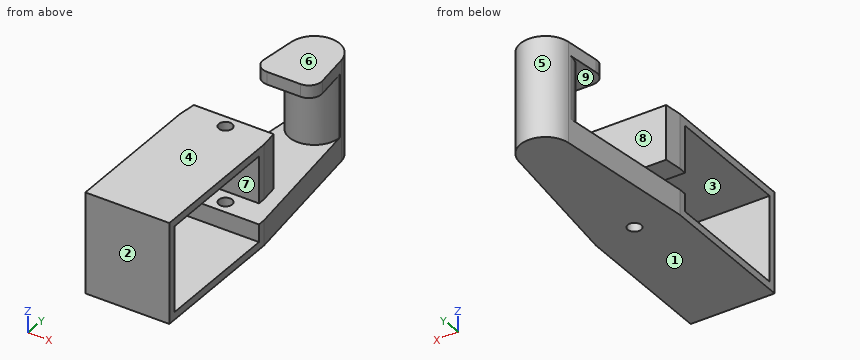
from build123d import *

# Parameters (mm, degrees)
EXTRUDE_1_DEPTH     = 24
CUT_EXTRUDE_1_DEPTH = 80.586658306
SKETCH_3_R          = 1.6
CUT_EXTRUDE_2_DEPTH = 80.586658306
CUT_EXTRUDE_3_DEPTH = 15
FILLET_1_R          = 3


with BuildPart() as part:
    # 草图1 → 凸台-拉伸1 (new body)
    with BuildSketch(Plane.XY):
        with BuildLine():
            Line((0, 0), (20, 0))
            Line((20, 0), (20, 34))
            Line((20, 34), (15.957817839, 67.908823654))
            ThreePointArc((15.957817839, 67.908823654), (10, 73.198607775), (4.042182161, 67.908823654))
            Line((4.042182161, 67.908823654), (0, 34))
            Line((0, 34), (0, 0))
        make_face()
    extrude(amount=EXTRUDE_1_DEPTH)

    # 草图2 → 切除-拉伸1 (cut, through all)
    with BuildSketch(Plane(origin=(20, 0, 0), x_dir=(0, 0, -1), z_dir=(1, 0, 0))):
        Polygon((-22.2, 32.2), (-11, 32.2), (-11, 38.2), (-24, 38.2), (-24, 56.198607775), (-21, 56.198607775), (-21, 61.198607775), (-6, 61.198607775), (-6, 38.2), (-6, 32.2), (-1.8, 32.2), (-1.8, 1.8), (-22.2, 1.8), align=None)
    extrude(amount=-CUT_EXTRUDE_1_DEPTH, mode=Mode.SUBTRACT)

    # 草图3 → 切除-拉伸2 (cut, through all)
    with BuildSketch(Plane.XY.offset(24)):
        with Locations((10, 35.269565603)):
            Circle(SKETCH_3_R)
    extrude(amount=-CUT_EXTRUDE_2_DEPTH, mode=Mode.SUBTRACT)

    # 草图4 → 切除-拉伸3 (cut)
    with BuildSketch(Plane.XY.offset(6)):
        with BuildLine():
            Line((16, 67.198607775), (19.499328987, 67.198607775))
            Line((19.499328987, 67.198607775), (19.499328987, 38.2))
            Line((19.499328987, 38.2), (0.500671013, 38.2))
            Line((0.500671013, 38.2), (0.500671013, 67.198607775))
            Line((0.500671013, 67.198607775), (4, 67.198607775))
            ThreePointArc((4, 67.198607775), (10, 61.198607775), (16, 67.198607775))
        make_face()
    extrude(amount=CUT_EXTRUDE_3_DEPTH, mode=Mode.SUBTRACT)

    # 圆角1
    fillet_1_edges = [part.edges().sort_by_distance(p)[0] for p in [
        (17.35376204, 56.198607775, 22.5),
        (2.64623796, 56.198607775, 22.5),
    ]]
    fillet(fillet_1_edges, radius=FILLET_1_R)


solid = part.part
Input: part model. Units: mm. Frame: model coordinates. Face numbers are marked on the shaded views. A direction names the side the tool comes from. Round coordinates to 2 decimals unless told otherwise and drop trailing zeros. Order: outer loops, then holes, each group sorted by start corner. A loop starts at its lowest first (then second) coordinate and runs counter-clockwise, first axis right, second up. Notation, with made-up numbers: (85, 66.25) - (93, 66.25) arc R13 ccw to (93, 70.25) - close; hole circle Ø11 at (70.5, 87.5). An arc over 180 degrees is marked (long way). Answer as a JSON object with one key per item and string values. Group by question number.
(1) Reachability of the marked faces 5, 6, 7, 8 and 9 from +Z, -Z, +X, -X, +Y, -Y: full face, straight path, thin tool, end or side. Return the list, or none.
(2) Cut plane A-A (y = 6). Return loops of the section in (x, z).
(3) Pin query (flat end, axial travel): P1, Ø6, axis at y = 38, z = 9, coming from the +X side; P2, Ø1.5, axis at x = 11.5, z = 17, coming from the +Y side. Return the tip coordinate at first contact, or that it passes through.
(4) Draft query along Z for the marked faces 1, 2, 3 and 4. Return one class per face: released by +Z, released by -Z, zero draft, split by the parting line, or undercut.
(5) Cut plane C-C (x = 10). Return loops of the section in (y, z), then the cut area to 3 significant figures.
(6) Cut plane D-D (z = 10.25). Return loops of the section in (x, y).
(7) Material intervals for probe 1 along Y at (x, z) = (10, 3.75); probe 2 along Y at (x, z) = (10, 14); probe 3 along Z at (x, y) = (4, 14.5), sorted ascending. Write a range as from..to.
(8) Cut plane B-B (z = 16). Return loops of the section in (x, y).
Here are the results:
{
 "1": {"face 5": "+Z, -Z, +Y", "face 6": "+Z, +X, -X, +Y, -Y", "face 7": "+X, -X", "face 8": "+Z, +X, -X", "face 9": "none"},
 "2": {"outline": "(0, 0) - (20, 0) - (20, 1.8) - (0, 1.8) - close; (0, 22.2) - (20, 22.2) - (20, 24) - (0, 24) - close"},
 "3": {"P1": "stops at x = 19.79", "P2": "stops at y = 73.15"},
 "4": {"face 1": "released by -Z", "face 2": "zero draft", "face 3": "undercut", "face 4": "released by +Z"},
 "5": {"outline": "(0, 0) - (33.67, 0) - (33.67, 6) - (32.2, 6) - (32.2, 1.8) - (1.8, 1.8) - (1.8, 22.2) - (32.2, 22.2) - (32.2, 11) - (33.67, 11) - (33.67, 24) - (0, 24) - close; (36.87, 0) - (73.2, 0) - (73.2, 24) - (56.2, 24) - (56.2, 21) - (61.2, 21) - (61.2, 6) - (36.87, 6) - close; (36.87, 11) - (38.2, 11) - (38.2, 24) - (36.87, 24) - close", "area": "647 mm^2"},
 "6": {"outline": "(0, 0) - (20, 0) - (20, 1.8) - (0, 1.8) - close; (3.96, 67.2) - (4, 67.2) arc R6 ccw to (16, 67.2) - (16.04, 67.2) - (15.96, 67.91) arc R6 ccw to (4.04, 67.91) - close"},
 "7": {"probe 1": "y = 0..1.8, 32.2..33.67, 36.87..73.2", "probe 2": "y = 0..1.8, 32.2..33.67, 36.87..38.2, 61.2..73.2", "probe 3": "z = 0..1.8, 22.2..24"},
 "8": {"outline": "(0, 0) - (20, 0) - (20, 1.8) - (0, 1.8) - close; (0, 32.2) - (20, 32.2) - (20, 34) - (19.5, 38.2) - (0.5, 38.2) - (0, 34) - close; (3.96, 67.2) - (4, 67.2) arc R6 ccw to (16, 67.2) - (16.04, 67.2) - (15.96, 67.91) arc R6 ccw to (4.04, 67.91) - close; hole circle Ø3.2 at (10, 35.27)"}
}
